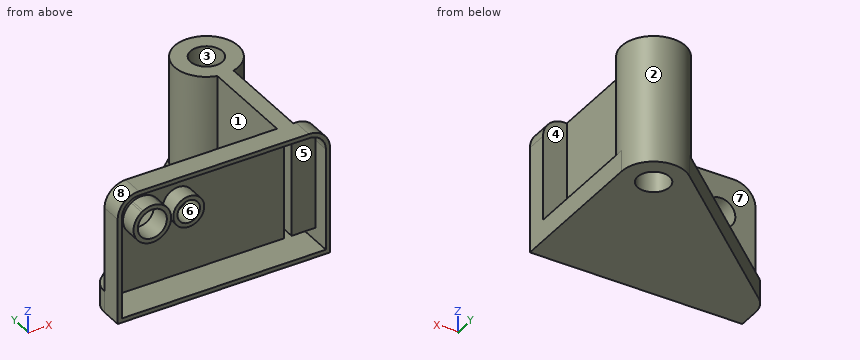
```python
from build123d import *

# Parameters (mm, degrees)
SKETCH1_W            = 127
SKETCH1_H            = 12.7
BOSS_EXTRUDE1_DEPTH  = 76.2
FILLET2_R            = 12.7
BOSS_EXTRUDE3_DEPTH  = 76.2
BOSS_EXTRUDE4_DEPTH  = 12.7
SKETCH3_R            = 8.693712638
SKETCH3_R_2          = 6.718686286
CUT_EXTRUDE2_DEPTH   = 177.090892723
SKETCH1_8_R          = 9.525
CUT_EXTRUDE3_DEPTH   = 159.75
SHELL4_START         = 2.54
SHELL4_OUTLINE_R     = 12.065
SHELL4_DEPTH         = 41.911304946
SHELL4_2_DEPTH       = 7.62
SHELL4_START_2       = 62.968677719
SHELL4_3_OUTLINE_R   = 12.065
SHELL4_3_DEPTH       = 0.531322281
SHELL4_START_3       = -50.8
SHELL4_4_DEPTH       = 10.16
SHELL4_START_4       = -40.64
SHELL4_5_OUTLINE_W   = 4.572
SHELL4_5_OUTLINE_H   = 18.517372773
SHELL4_5_OUTLINE_H_2 = 10.16
SHELL4_5_DEPTH       = 66.6749999
SHELL4_6_DEPTH       = 10.16
SHELL4_START_5       = 44.451304946
SHELL4_7_OUTLINE_R   = 12.065
SHELL4_7_DEPTH       = 29.208695054


with BuildPart() as part:
    # Sketch1 → Boss-Extrude1 (new body)
    with BuildSketch(Plane.XY):
        with Locations((-63.5, -44.45)):
            Rectangle(SKETCH1_W, SKETCH1_H)
    extrude(amount=BOSS_EXTRUDE1_DEPTH)

    # Fillet2
    fillet2_edges = [part.edges().sort_by_distance(p)[0] for p in [
        (-127, -44.45, 76.2),
        (0, -44.45, 76.2),
    ]]
    fillet(fillet2_edges, radius=FILLET2_R)

    # Sketch1<6> → Boss-Extrude3 (add)
    with BuildSketch(Plane.XY):
        with BuildLine():
            ThreePointArc((-14.224, 19.671429138), (-19.05, 57.15), (-23.876, 19.671429138))
            Line((-23.876, 19.671429138), (-23.876, -38.1))
            Line((-23.876, -38.1), (-14.224, -38.1))
            Line((-14.224, -38.1), (-14.224, 19.671429138))
        make_face()
    extrude(amount=BOSS_EXTRUDE3_DEPTH)

    # Sketch1<7> → Boss-Extrude4 (add)
    with BuildSketch(Plane.XY):
        with BuildLine():
            ThreePointArc((-23.876, 19.671429138), (-37.59378257, 33.737589198), (-31.585775702, 52.444226279))
            Line((-31.585775702, 52.444226279), (-122.686278821, -27.170766624))
            ThreePointArc((-122.686278821, -27.170766624), (-125.882553095, -32.225131223), (-127, -38.1))
            Line((-127, -38.1), (-23.876, -38.1))
            Line((-23.876, -38.1), (-23.876, 19.671429138))
        make_face()
        with BuildLine():
            Line((0, -38.1), (0, 38.1))
            ThreePointArc((0, 38.1), (-3.969585549, 26.460257735), (-14.224, 19.671429138))
            Line((-14.224, 19.671429138), (-14.224, -38.1))
            Line((-14.224, -38.1), (0, -38.1))
        make_face()
    extrude(amount=BOSS_EXTRUDE4_DEPTH)

    # Sketch3 → Cut-Extrude2 (cut, through all)
    with BuildSketch(Plane(origin=(0, -38.1, 0), x_dir=(1, 0, 0), z_dir=(0, 1, 0))):
        with Locations(Location((-106.276718745, -53.709991333, 0), (0, 0, 180))):
            Circle(SKETCH3_R)
        with Locations(Location((-84.500771906, -53.709991333, 0), (0, 0, 180))):
            Circle(SKETCH3_R_2)
    extrude(amount=-CUT_EXTRUDE2_DEPTH, mode=Mode.SUBTRACT)

    # Sketch1<8> → Cut-Extrude3 (cut, through all)
    with BuildSketch(Plane.XY):
        with Locations((-19.05, 38.1)):
            Circle(SKETCH1_8_R)
    extrude(amount=CUT_EXTRUDE3_DEPTH, mode=Mode.SUBTRACT)

    # Shell4: read off the stored shape, not the designer's step
    # Shell4 outline → Shell4 (cut)
    with BuildSketch(Plane.XY.offset(SHELL4_START)):
        with BuildLine():
            ThreePointArc((-16.764, 21.74902743), (-19.05, 54.61), (-21.336, 21.74902743))
            Line((-21.336, 21.74902743), (-21.336, -40.64))
            Line((-21.336, -40.64), (-124.46, -40.64))
            Line((-124.46, -40.64), (-124.46, -50.8))
            Line((-124.46, -50.8), (-2.54, -50.8))
            Line((-2.54, -50.8), (-2.54, -40.64))
            Line((-2.54, -40.64), (-16.764, -40.64))
            Line((-16.764, -40.64), (-16.764, 21.74902743))
        make_face()
        with Locations((-19.05, 38.1)):
            Circle(SHELL4_OUTLINE_R, mode=Mode.SUBTRACT)
    extrude(amount=SHELL4_DEPTH, mode=Mode.SUBTRACT)

    # Shell4 2 outline → Shell4 2 (cut)
    with BuildSketch(Plane.XY.offset(SHELL4_START)):
        with BuildLine():
            Line((-21.336, -40.64), (-21.336, 21.74902743))
            ThreePointArc((-21.336, 21.74902743), (-34.872227338, 33.384364087), (-29.914338942, 50.531662775))
            Line((-29.914338942, 50.531662775), (-120.914264565, -28.995432955))
            ThreePointArc((-120.914264565, -28.995432955), (-123.542285503, -33.214680644), (-124.46, -38.1))
            Line((-124.46, -38.1), (-124.46, -40.64))
            Line((-124.46, -40.64), (-21.336, -40.64))
        make_face()
        with BuildLine():
            Line((-2.54, -40.64), (-2.54, 38.1))
            ThreePointArc((-2.54, 38.1), (-6.593636968, 27.263989664), (-16.764, 21.74902743))
            Line((-16.764, 21.74902743), (-16.764, -40.64))
            Line((-16.764, -40.64), (-2.54, -40.64))
        make_face()
    extrude(amount=SHELL4_2_DEPTH, mode=Mode.SUBTRACT)

    # Shell4 3 outline → Shell4 3 (cut)
    with BuildSketch(Plane.XY.offset(SHELL4_START_2)):
        with BuildLine():
            ThreePointArc((-16.764, 21.74902743), (-19.05, 54.61), (-21.336, 21.74902743))
            Line((-21.336, 21.74902743), (-21.336, -40.64))
            Line((-21.336, -40.64), (-124.46, -40.64))
            Line((-124.46, -40.64), (-124.46, -50.8))
            Line((-124.46, -50.8), (-2.54, -50.8))
            Line((-2.54, -50.8), (-2.54, -40.64))
            Line((-2.54, -40.64), (-16.764, -40.64))
            Line((-16.764, -40.64), (-16.764, 21.74902743))
        make_face()
        with Locations((-19.05, 38.1)):
            Circle(SHELL4_3_OUTLINE_R, mode=Mode.SUBTRACT)
    extrude(amount=SHELL4_3_DEPTH, mode=Mode.SUBTRACT)

    # Shell4 4 outline → Shell4 4 (cut)
    with BuildSketch(Plane(origin=(0, 0, 0), x_dir=(1, 0, 0), z_dir=(0, 1, 0)).offset(SHELL4_START_3)):
        with BuildLine():
            Line((-2.54, -62.968677719), (-2.54, -44.451304946))
            Line((-2.54, -44.451304946), (-84.500771906, -44.451305047))
            ThreePointArc((-84.500771906, -44.451305047), (-75.24208562, -53.709991333), (-84.500771906, -62.968677619))
            Line((-84.500771906, -62.968677619), (-2.54, -62.968677719))
        make_face()
        with BuildLine():
            ThreePointArc((-12.7, -73.66), (-5.515795103, -70.684204897), (-2.54, -63.5))
            Line((-2.54, -63.5), (-100.767451105, -63.5))
            ThreePointArc((-100.767451105, -63.5), (-106.276718745, -64.943703971), (-111.785986385, -63.5))
            Line((-111.785986385, -63.5), (-124.46, -63.5))
            ThreePointArc((-124.46, -63.5), (-121.484204897, -70.684204897), (-114.3, -73.66))
            Line((-114.3, -73.66), (-12.7, -73.66))
        make_face()
        with BuildLine():
            ThreePointArc((-84.500771906, -62.968677619), (-93.759458192, -53.709991333), (-84.500771906, -44.451305047))
            Line((-84.500771906, -44.451305047), (-99.914877343, -44.451304946))
            ThreePointArc((-99.914877343, -44.451304946), (-95.043006107, -53.709991332), (-99.914877342, -62.968677719))
            Line((-99.914877342, -62.968677719), (-84.500771906, -62.968677619))
        make_face()
        with BuildLine():
            ThreePointArc((-112.638560148, -62.968677719), (-117.510431383, -53.709991332), (-112.638560147, -44.451304946))
            Line((-112.638560147, -44.451304946), (-124.46, -44.451304946))
            Line((-124.46, -44.451304946), (-124.46, -62.968677719))
            Line((-124.46, -62.968677719), (-112.638560148, -62.968677719))
        make_face()
    extrude(amount=SHELL4_4_DEPTH, mode=Mode.SUBTRACT)

    # Shell4 5 outline → Shell4 5 (cut)
    with BuildSketch(Plane(origin=(0, 0, 0), x_dir=(1, 0, 0), z_dir=(0, 1, 0)).offset(SHELL4_START_4)):
        with Locations((-19.05, -53.709991333)):
            Rectangle(SHELL4_5_OUTLINE_W, SHELL4_5_OUTLINE_H)
        with Locations((-19.05, -68.58)):
            Rectangle(SHELL4_5_OUTLINE_W, SHELL4_5_OUTLINE_H_2)
    extrude(amount=SHELL4_5_DEPTH, mode=Mode.SUBTRACT)

    # Shell4 6 outline → Shell4 6 (add)
    with BuildSketch(Plane(origin=(0, 0, 0), x_dir=(1, 0, 0), z_dir=(0, 1, 0)).offset(SHELL4_START_3)):
        with BuildLine():
            Line((-112.638560147, -44.451304946), (-99.914877343, -44.451304946))
            ThreePointArc((-99.914877343, -44.451304946), (-106.276718745, -42.476278695), (-112.638560147, -44.451304946))
        make_face()
        with BuildLine():
            Line((-111.785986385, -63.5), (-100.767451105, -63.5))
            ThreePointArc((-100.767451105, -63.5), (-100.335222021, -63.243873874), (-99.914877342, -62.968677719))
            Line((-99.914877342, -62.968677719), (-112.638560148, -62.968677719))
            ThreePointArc((-112.638560148, -62.968677719), (-112.218215469, -63.243873874), (-111.785986385, -63.5))
        make_face()
    extrude(amount=SHELL4_6_DEPTH)

    # Shell4 7 outline → Shell4 7 (cut)
    with BuildSketch(Plane.XY.offset(SHELL4_START_5)):
        with BuildLine():
            ThreePointArc((-16.764, 21.74902743), (-19.05, 54.61), (-21.336, 21.74902743))
            Line((-21.336, 21.74902743), (-19.05, 21.429425891))
            Line((-19.05, 21.429425891), (-16.764, 21.74902743))
        make_face()
        with Locations((-19.05, 38.1)):
            Circle(SHELL4_7_OUTLINE_R, mode=Mode.SUBTRACT)
    extrude(amount=SHELL4_7_DEPTH, mode=Mode.SUBTRACT)


solid = part.part
```
Model file for the job. Use its own axes, mm. Face numbers are marked on the shaded views. A direction names the side the tool comes from. Coordinates: 2 decimals unless noted, no trailing zeros. Write each loop counter-clockwise with the first axis right and the second up, starting at its lowest first coordinate (ties: lowest second). Pieces come first, ordered by that corner, then holes. Notation, with made-up numbers: (87, -14) - (114, -14) arc R24 ccw to (114, 15) - close; hole circle Ø9 at (77, 23.25). An arc over 180 degrees is marked (long way). One line per item, written item: value. Start each with the question number.
1. Slice it at B-B (y = 44). Write the cut outline in (x, z).
2. Tool access for the marked faces 1, 2, 3, 4 and 5: list every direction of +Z, -Z, +X, -X, +Y, -Y with a clear straight run to the whole face (end or side of a thin tool).
3. Flat gauge pins, fed straight in: pin 1 (17.5 mm diameter, centred on x = -84.5, z = 53.71, fed in from +Y); pin 2 (1 mm diameter, centred on x = -97.5, y = -5, fed in from -Z); pin 3 (10 mm diameter, centred on y = -10, z = 39.5, fed in from +X); pin 4 (7 mm diameter, centred on x = -9, z = 41.5, fed in from -Y). Where does each tip first touch, or does it go through?
4. Slice it at D-D (x = -46). Write the cut outline in (y, z), plus the area to 3 significant figures.
5. Slice it at C-C (y = -5). Write the cut outline in (x, z).
6. Mould opens along Z. For the marked faces 6, 7 and 8 say: released by +Z, released by -Z, zero draft, split by the parting line, or undercut.
7. Probe line 1 (Y direction, x = -19.05, z = 52) (3 decimals); line 2 (Z direction, x = -67, y = -27.5); line 3 (X direction, y = -8.5, z = 69). List the from-to ranges inside material, lowest first. Write a range as from..to.
8. Slice it at A-A (x = -19.05). Write the cut outline in (y, z) (3 decimals).
Answers below:
1. outline: (-41.25, 0) - (-26.53, 0) - (-26.53, 76.2) - (-37.16, 76.2) - (-37.16, 12.7) - (-41.25, 12.7) - close; (-11.57, 0) - (-0.94, 0) - (-0.94, 76.2) - (-11.57, 76.2) - close; hole (-37.39, 2.54) - (-29.57, 2.54) - (-29.57, 73.66) - (-34.47, 73.66) - (-34.47, 10.16) - (-37.39, 10.16) - close; hole (-8.53, 2.54) - (-3.63, 2.54) - (-3.63, 73.66) - (-8.53, 73.66) - close
2. face 1: +Z, -X
2. face 2: +Z
2. face 3: +Z, -Z
2. face 4: +Z, +X
2. face 5: -Y
3. pin 1: stops at y = -38.1
3. pin 2: stops at z = 0
3. pin 3: stops at x = -14.22
3. pin 4: stops at y = -40.64
4. outline: (-50.8, 0) - (39.85, 0) - (39.85, 12.7) - (-38.1, 12.7) - (-38.1, 76.2) - (-50.8, 76.2) - (-50.8, 73.66) - (-40.64, 73.66) - (-40.64, 10.16) - (36.47, 10.16) - (36.47, 2.54) - (-50.8, 2.54) - close
4. area: 647 mm^2
5. outline: (-97.32, 0) - (0, 0) - (0, 12.7) - (-14.22, 12.7) - (-14.22, 76.2) - (-23.88, 76.2) - (-23.88, 12.7) - (-97.32, 12.7) - close; hole (-93.46, 2.54) - (-2.54, 2.54) - (-2.54, 10.16) - (-16.76, 10.16) - (-16.76, 73.66) - (-21.34, 73.66) - (-21.34, 10.16) - (-93.46, 10.16) - close
6. face 6: undercut
6. face 7: zero draft
6. face 8: released by +Z
7. line 1: y = 26.035..28.575, 47.625..50.165, 54.61..57.15
7. line 2: z = 0..2.54, 10.16..12.7
7. line 3: x = -23.88..-21.34, -16.76..-14.22
8. outline: (-50.8, 0) - (28.575, 0) - (28.575, 76.2) - (-50.8, 76.2) - (-50.8, 73.66) - (26.035, 73.66) - (26.035, 2.54) - (-50.8, 2.54) - close; (47.625, 0) - (57.15, 0) - (57.15, 76.2) - (47.625, 76.2) - close; hole (50.165, 2.54) - (54.61, 2.54) - (54.61, 73.66) - (50.165, 73.66) - close
